```python
from build123d import *

# Parameters (mm, degrees)
F0_W     = 28
F0_H     = 28
F1_DEPTH = 24
F2_R     = 12
F3_DEPTH = 20
F4_R     = 1
F5_DEPTH = 2
F6_W     = 5
F6_H     = 6
F7_DEPTH = 8


with BuildPart() as f1:
    # F0 (on Top) → F1 (new body)
    with BuildSketch(Plane.XY):
        Rectangle(F0_W, F0_H)
    extrude(amount=F1_DEPTH)

    # F2 (on face) → F3 (cut)
    with BuildSketch(Plane.XY.offset(24)):
        Circle(F2_R)
    extrude(amount=-F3_DEPTH, mode=Mode.SUBTRACT)

    # F4 (on face) → F5 (join)
    with BuildSketch(Plane.XY.offset(24)):
        with Locations((-11, 11)):
            Circle(F4_R)
        with Locations((11, 11)):
            Circle(F4_R)
        with Locations((11, -11)):
            Circle(F4_R)
        with Locations((-11, -11)):
            Circle(F4_R)
    extrude(amount=F5_DEPTH)

    # F6 (on face) → F7 (cut)
    with BuildSketch(Plane.XY.offset(24)):
        with Locations((-10.5, 6)):
            Rectangle(F6_W, F6_H)
        with Locations((10.5, -6)):
            Rectangle(F6_W, F6_H)
    extrude(amount=-F7_DEPTH, mode=Mode.SUBTRACT)


solid = f1.part
```
Can you work these out from the model? Positions are in its coordinate system, mm. A direction names the side the tool comes from. Give positions to 0.01 mm unless a question says otherwise; leave off trailing zeros. Loops run counter-clockwise (first coordinate to the right, second up) from the corner with the lowest first, then second, coordinate; pieces in that order, holes last. Notation, with made-up numbers: M -2.75,2.25 L 15.25,2.25 A15 cw 15.25,23.25 Z; hole C 29,-34.5 d8. An arc over 180 degrees is marked long. One line per item, written item: value.
(1) Suppose I cut it at A-A on x = -3. List the corners of the cut face in (y, z) for me.
Returned:
outline: M -14,0 L 14,0 L 14,24 L 11.62,24 L 11.62,4 L -11.62,4 L -11.62,24 L -14,24 Z
(2) Will these pins go through, and if not, where does the flat tip stop? pin 1 (6 mm diameter, centred on x = -9, y = 1.5, fed in from +Z); pin 2 (12 mm diameter, centred on x = 1, y = 3.5, fed in from +Z); pin 3 (2.5 mm diameter, centred on x = 9.5, y = -6, fed in from +Z).
Returned:
pin 1: z = 24
pin 2: z = 4
pin 3: z = 16
(3) I need wall thicknesses on line 1 (X direction, y = 0, z = 19.5); line 2 (Y direction, x = -12.25, z = 16.5). Which ranges of each line are inside material? Lowest first, please.
Returned:
line 1: -14 to -12, 12 to 14
line 2: -14 to 3, 9 to 14
(4) We'd pull the mould along Y, two halves only. Please class faces 1 (the face through (-11, -11, 26)), 2 (the face through (12, -7, 16)), 3 (the face through (0, -14, 12)): released by +Y, released by -Y, zero draft, split by the parting line, or undercut.
Returned:
face 1: zero draft
face 2: undercut
face 3: released by -Y
(5) Suppose I cut it at B-B on z = 22.75. List the corners of the cut face in (x, y) for me.
Returned:
outline: M -14,-14 L 14,-14 L 14,14 L -14,14 Z; hole M -13,3 L -11.62,3 A12 ccw 8,-8.94 L 8,-9 L 13,-9 L 13,-3 L 11.62,-3 A12 ccw -8,8.94 L -8,9 L -13,9 Z
(6) Which directions (+Z, -Z, +X, -X, +Y, -Y) give clear straight access to the entire face, cutting with the end or side of a thin tool? Please do faces 4 (the face through (11, -11, 26)), 5 (the face through (12, -3, 20)).
Returned:
face 4: +Z, +X, -X, +Y, -Y
face 5: +Z
(7) Suppose I cut it at D-D on y = 11.5. List the corners of the cut face in (x, z) for me, plus the area to 3 significant figures.
Returned:
outline: M -14,0 L 14,0 L 14,24 L 11.87,24 L 11.87,26 L 10.13,26 L 10.13,24 L 3.43,24 L 3.43,4 L -3.43,4 L -3.43,24 L -10.13,24 L -10.13,26 L -11.87,26 L -11.87,24 L -14,24 Z
area: 542 mm^2
(8) Suppose I cut it at C-C on y = 0. List the corners of the cut face in (x, z) for me.
Returned:
outline: M -14,0 L 14,0 L 14,24 L 12,24 L 12,4 L -12,4 L -12,24 L -14,24 Z
